Work out the finished part from the listing and answer in its coordinate system (mm). Give positions to 0.01 mm unless a question says otherwise; leave off trailing zeros. Loops run counter-clockwise (first coordinate to the right, second up) from the corner with the lowest first, then second, coordinate; pieces in that order, holes last. Notation, with made-up numbers: (89.5, -32.5) -> (121.5, -32.5) arc R18 ccw to (121.5, -10.5) -> close; hole circle Ø2 at (69, 22). An arc over 180 degrees is marked (long way). Answer as CSV lines item,"result". Start each with the question number.
1. Find section B-B, the plane y = 0.5. Give the vertices of the cut face in (x, z), and give its area (3 significant figures).
2. Find section C-C, the plane x = 21.59. Give the vertices of the cut face in (y, z), and give its area (3 significant figures).
3. Find section D-D, the plane x = -41.91. Give the vertices of the cut face in (y, z), and give its area (3 significant figures).
4. Find section A-A, the plane z = 0. Give the vertices of the cut face in (x, y).
5. Find the intervals of material crossed by line 1 along Z through (x, y) = (-41.91, 0.65); line 2 along Z through (x, y) = (-21.5, 0.2); line 3 along Z through (x, y) = (29.5, 0.65), in increasing order.
6. Flat-ended cylindrical pins translate along their axes: pin 1 Ø2 at (x, z) = (-41.91, 0) entering from +Y; pin 2 Ø3.5 at (x, z) = (-21.59, 0) entering from +Y. Find the tip coordinate at first contact, or state that the pin passes through.
Autodesk Inventor part; units mm, degrees
ref_plane "YZ Plane" through (0, 0, 0) normal (1, 0, 0) x (0, 1, 0)
ref_plane "XZ Plane" through (0, 0, 0) normal (0, 1, 0) x (-1, 0, 0)
ref_plane "XY Plane" through (0, 0, 0) normal (0, 0, 1) x (1, 0, 0)
sketch "Sketch1" plane through (0, 0, 0) normal (0, 1, 0) x (-1, 0, 0)
  line L0 (44.45, 31.7246) -> (44.45, -31.7246)
  line L1 (-44.45, -31.7246) -> (-44.45, 31.7246)
  arc A0 (-44.45, -31.7246) -> (44.45, -31.7246) centre (0, 0) ccw
  arc A1 (44.45, 31.7246) -> (-44.45, 31.7246) centre (0, 0) ccw
  line L2 (44.45, 0) -> (41.91, 0)
  circle A2 centre (41.91, 0) radius 1.27
  line L3 (41.91, 0) -> (21.59, 0)
  circle A3 centre (21.59, 0) radius 1.27
  line L4 (0, -54.61) -> (0, 54.61)
  circle A4 centre (-41.91, 0) radius 1.27
  circle A5 centre (-21.59, 0) radius 1.27
  dimension "d3" = 88.9
  dimension "d4" = 2.54
  dimension "d5" = 2.54
  dimension "d6" = 20.32
  dimension "d7" = 2.54
extrude "Extrusion1" add sketch "Sketch1" along normal blind 2.032
properties part number "Top Plate"
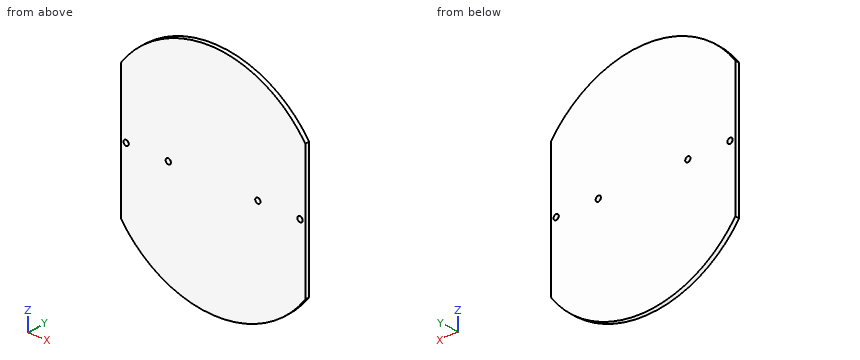
Resolved:
1,outline,"(-44.45, -31.72) arc R54.61 ccw to (44.45, -31.72) -> (44.45, 31.72) arc R54.61 ccw to (-44.45, 31.72) -> close; hole circle Ø2.54 at (-41.91, 0); hole circle Ø2.54 at (-21.59, 0); hole circle Ø2.54 at (21.59, 0); hole circle Ø2.54 at (41.91, 0)"
1,area,"8,470 mm^2"
2,outline,"(0, -50.16) -> (2.03, -50.16) -> (2.03, -1.27) -> (0, -1.27) -> close; (0, 1.27) -> (2.03, 1.27) -> (2.03, 50.16) -> (0, 50.16) -> close"
2,area,"199 mm^2"
3,outline,"(0, -35.01) -> (2.03, -35.01) -> (2.03, -1.27) -> (0, -1.27) -> close; (0, 1.27) -> (2.03, 1.27) -> (2.03, 35.01) -> (0, 35.01) -> close"
3,area,"137 mm^2"
4,outline,"(-44.45, 0) -> (-43.18, 0) -> (-43.18, 2.03) -> (-44.45, 2.03) -> close; (-40.64, 0) -> (-22.86, 0) -> (-22.86, 2.03) -> (-40.64, 2.03) -> close; (-20.32, 0) -> (20.32, 0) -> (20.32, 2.03) -> (-20.32, 2.03) -> close; (22.86, 0) -> (40.64, 0) -> (40.64, 2.03) -> (22.86, 2.03) -> close; (43.18, 0) -> (44.45, 0) -> (44.45, 2.03) -> (43.18, 2.03) -> close"
5,line 1,"z = -35.01 to -1.27, 1.27 to 35.01"
5,line 2,"z = -50.2 to -1.27, 1.27 to 50.2"
5,line 3,"z = -45.96 to 45.96"
6,pin 1,"passes through"
6,pin 2,"stops at y = 2.03"
